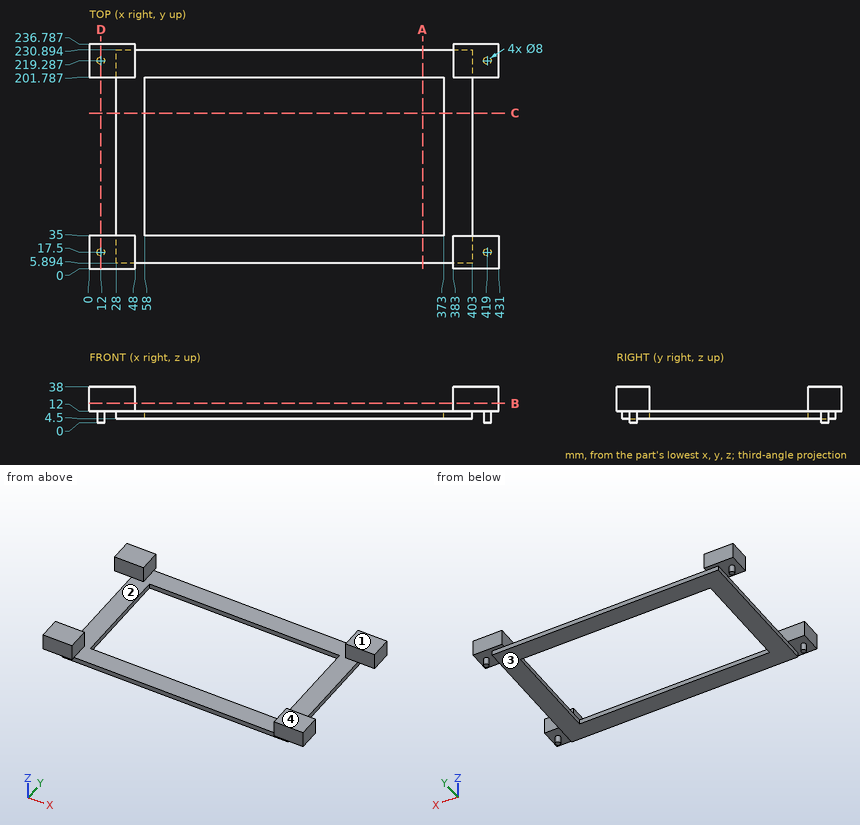
Answer from the drawing. Dimensions are ordinates in mm from the lowest x, y and z of the part. A direction names the side the tool comes from. Give positions to 0.01 mm unless a question says otherwise; leave off trailing zeros. Order: outer loops, then holes, each group sorted by start corner. A loop starts at its lowest first (then second) coordinate and runs counter-clockwise, first axis right, second up.
Item 1: The part is cut by section C-C, the plane y = 164. Give the vertices of the cut face in (x, z), and give its area (3 significant figures).
From the geometry:
outline: (28, 4.5) - (58, 4.5) - (58, 12) - (28, 12) - close; (373, 4.5) - (403, 4.5) - (403, 12) - (373, 12) - close
area: 450 mm2
Item 2: Which of the six approach directions +Z, -Z, +X, -X, +Y, -Y give full straight-line access (tool end or side, diameter ignored) to the marked faces 3 and 4?
From the geometry:
face 3: -Z, +Y, -Y
face 4: +Z, +X, -X, +Y, -Y
Item 3: For a pull along Y with two mould halves and no side action, classify the marked faces 1 and 2 as pulls with the +Y half, pulls with the -Y half, needs draft (parallel to the pull), parting line crosses it, or undercut.
From the geometry:
face 1: needs draft
face 2: undercut
Item 4: The part is cut by section D-D, the plane x = 12. Give the vertices of the cut face in (y, z).
From the geometry:
outline: (0, 12) - (13.5, 12) - (13.5, 0) - (21.5, 0) - (21.5, 12) - (35, 12) - (35, 38) - (0, 38) - close; (201.79, 12) - (215.29, 12) - (215.29, 0) - (223.29, 0) - (223.29, 12) - (236.79, 12) - (236.79, 38) - (201.79, 38) - close
Item 5: Find the intervals of material crossed by probe 1 along X at (y, z) = (182.5, 11.5); probe 2 along X at (y, z) = (22.5, 32); probe 3 along Y at (x, z) = (359.5, 6), in increasing order.
From the geometry:
probe 1: x = 28 to 58, 373 to 403
probe 2: x = 0 to 48, 383 to 431
probe 3: y = 5.89 to 35, 201.79 to 230.89
Item 6: The part is cut by section B-B, the plane z = 20.5. Give the vertices of the cut face in (x, y).
From the geometry:
outline: (0, 0) - (48, 0) - (48, 35) - (0, 35) - close; (0, 201.79) - (48, 201.79) - (48, 236.79) - (0, 236.79) - close; (383, 0) - (431, 0) - (431, 35) - (383, 35) - close; (383, 201.79) - (431, 201.79) - (431, 236.79) - (383, 236.79) - close
Item 7: The part is cut by section A-A, the plane x = 351. Give the vertices of the cut face in (y, z).
From the geometry:
outline: (5.89, 4.5) - (35, 4.5) - (35, 12) - (5.89, 12) - close; (201.79, 4.5) - (230.89, 4.5) - (230.89, 12) - (201.79, 12) - close
Item 8: Given pin 1 Ø4 at (y, z) = (114.5, 10) entering from -X; pin 2 Ø6 at (x, y) = (182, 207) entering from -Z; pin 3 Ø6 at (x, y) = (291.5, 209) entering from +Z, each flat-ended and moving along its own axis, determine where each tip first touches the part or whether it passes through.
From the geometry:
pin 1: stops at x = 28
pin 2: stops at z = 4.5
pin 3: stops at z = 12
